Model file for the job. Use its own axes, mm. A direction names the side the tool comes from. Round coordinates to 2 decimals unless told otherwise and drop trailing zeros. Order: outer loops, then holes, each group sorted by start corner. A loop starts at its lowest first (then second) coordinate and runs counter-clockwise, first axis right, second up. Notation, with made-up numbers: (45.25, 57.5) -> (80.25, 57.5) arc R25 ccw to (80.25, 73.5) -> close; hole circle Ø10 at (66.25, -36.5). An arc over 180 degrees is marked (long way). Put each result on its own line as item: value. Start each with the question number.
Q1. 3-axis set-ups, long thin cutter, end or side, ignore diameter. For faces 5 (the face through (-6.4, 0, 0)), 6 (the face through (0, 1, 2.9)), 7 (the face through (5, -3.15, 0)), 8 (the face through (0, -3.15, 0)): which of +Z, -Z, +X, -X, +Y, -Y reach the whole face in a straight line?
Q2. Cut at D-D, the plane x = 3.25. List the corners of the cut face in (y, z).
Q3. Probe L1, parallel to Y at x = -3.25, z = 0.4; L2, parallel to Y at x = 3.25, z = -0.15; L3, parallel to X at y = 1, z = -2.15. List the from-to ranges inside material, lowest first.
Q4. Cut at C-C, the plane x = -2. List the corners of the cut face in (y, z).
Q5. Pull direction Y, two halves, no side cores. Call faces 1 (the face through (-1.62, 4.63, 0.02)), 2 (the face through (-3.987, -1.474, 0.041)), 3 (the face through (0, 1, -2.9)), 4 (the face through (-5, -3.15, 0)): released by +Y, released by -Y, zero draft, split by the parting line, or undercut.
Q6. Flat gauge pins, fed straight in: P1, Ø1.5, axis at y = -2.5, z = 1, coming from the -X side; P2, Ø1, axis at x = -1.5, z = -2, coming from the +Y side; P3, Ø1.3, axis at x = 4.5, z = -0.5, coming from the -Y side; P4, Ø2.5, axis at x = 3.25, y = -2.15, coming from the -Z side. Where does each tip first touch, or does it go through?
Q7. Cut at A-A, the plane z = 0. List the corners of the cut face in (x, y) (3 decimals), and give its area (3 significant figures).
Q8. Cut at B-B, the plane y = -2.15. List the corners of the cut face in (x, z), and give its area (3 significant figures).
from build123d import *

# Parameters (mm, degrees)
SKETCH1_W           = 12.8
SKETCH1_H           = 6.3
BOSS_EXTRUDE1_DEPTH = 2.9
BOSS_EXTRUDE3_DEPTH = 5.8
SKETCH2_3_R         = 1
CUT_EXTRUDE2_DEPTH  = 10.376699846
EXTRUDE_THIN1_DEPTH = 1.6


with BuildPart() as part:
    # Sketch1 → Boss-Extrude1 (new, symmetric)
    with BuildSketch(Plane.XY):
        Rectangle(SKETCH1_W, SKETCH1_H)
    extrude(amount=BOSS_EXTRUDE1_DEPTH, both=True)

    # Sketch2 → Boss-Extrude3 (add, through all)
    with BuildSketch(Plane.XY.offset(2.9)):
        Polygon((-4.508746523, -1.958141571), (-3.531951604, -0.266283143), (-1.578361765, -0.266283143), (-0.601566846, -1.958141571), (-1.578361765, -3.65), (-3.531951604, -3.65), align=None)
        Polygon((3.531951604, -0.266283143), (1.578361765, -0.266283143), (0.601566846, -1.958141571), (1.578361765, -3.65), (3.531951604, -3.65), (4.508746523, -1.958141571), align=None)
    extrude(amount=-BOSS_EXTRUDE3_DEPTH)

    # Sketch2<3> → Cut-Extrude2 (cut, through all)
    with BuildSketch(Plane.XY.offset(2.9)):
        with Locations((3.25, -2.15)):
            Circle(SKETCH2_3_R)
        with Locations((-3.25, -2.15)):
            Circle(SKETCH2_3_R)
    extrude(amount=-CUT_EXTRUDE2_DEPTH, mode=Mode.SUBTRACT)

    # Sketch3 → Extrude-Thin1 (add, symmetric)
    with BuildSketch(Plane.XY):
        Polygon((5.425, 3.15), (5.425, 3.502848465), (-8.175922459, 6.17265917), (-8.224077541, 5.92734083), (5.175, 3.297151535), (5.175, 3.15), align=None)
    extrude(amount=EXTRUDE_THIN1_DEPTH, both=True)


solid = part.part
Ans:
1. face 5: +Z, -Z, -X, -Y
1. face 6: +Z, +X, -X, +Y, -Y
1. face 7: +Z, -Z, +X, -Y
1. face 8: +Z, -Z, -Y
2. outline: (-3.65, -2.9) -> (-3.15, -2.9) -> (-3.15, 2.9) -> (-3.65, 2.9) -> close; (-1.15, -2.9) -> (3.15, -2.9) -> (3.15, 2.9) -> (-1.15, 2.9) -> close; (3.68, -1.6) -> (3.93, -1.6) -> (3.93, 1.6) -> (3.68, 1.6) -> close
3. L1: y = -3.65 to -3.15, -1.15 to 3.15, 4.95 to 5.21
3. L2: y = -3.65 to -3.15, -1.15 to 3.15, 3.68 to 3.93
3. L3: x = -6.4 to 6.4
4. outline: (-3.65, -2.9) -> (3.15, -2.9) -> (3.15, 2.9) -> (-3.65, 2.9) -> close; (4.71, -1.6) -> (4.96, -1.6) -> (4.96, 1.6) -> (4.71, 1.6) -> close
5. face 1: undercut
5. face 2: undercut
5. face 3: zero draft
5. face 4: released by -Y
6. P1: stops at x = -6.4
6. P2: stops at y = 4.92
6. P3: stops at y = -3.15
6. P4: stops at z = -2.9
7. outline: (-8.224, 5.927) -> (5.175, 3.297) -> (5.175, 3.15) -> (-6.4, 3.15) -> (-6.4, -3.15) -> (-3.821, -3.15) -> (-3.532, -3.65) -> (-1.578, -3.65) -> (-1.29, -3.15) -> (1.29, -3.15) -> (1.578, -3.65) -> (3.532, -3.65) -> (3.821, -3.15) -> (6.4, -3.15) -> (6.4, 3.15) -> (5.425, 3.15) -> (5.425, 3.503) -> (-8.176, 6.173) -> close; hole circle Ø2 at (-3.25, -2.15); hole circle Ø2 at (3.25, -2.15)
7. area: 80.1 mm^2
8. outline: (-6.4, -2.9) -> (-4.25, -2.9) -> (-4.25, 2.9) -> (-6.4, 2.9) -> close; (-2.25, -2.9) -> (2.25, -2.9) -> (2.25, 2.9) -> (-2.25, 2.9) -> close; (4.25, -2.9) -> (6.4, -2.9) -> (6.4, 2.9) -> (4.25, 2.9) -> close
8. area: 51.0 mm^2
